from build123d import *

# Parameters (mm, degrees)
BOSS_EXTRUDE1_DEPTH = 6


with BuildPart() as part:
    # Sketch1 → Boss-Extrude1 (new body)
    with BuildSketch(Plane(origin=(330, 0, 0), x_dir=(0, 0, -1), z_dir=(1, 0, 0))):
        Polygon((-52.75, 244), (-52.75, 250), (-78.625, 250), (-78.625, 244), (-105, 244), (-105, 6), (-78.625, 6), (-78.625, 0), (-52.75, 0), (-52.75, 6), (-25.875, 6), (-25.875, 0), (0, 0), (0, 22.272727273), (-6, 22.272727273), (-6, 45.545454545), (0, 45.545454545), (0, 67.818181818), (-6, 67.818181818), (-6, 91.090909091), (0, 91.090909091), (0, 113.363636364), (-6, 113.363636364), (-6, 136.636363636), (0, 136.636363636), (0, 158.909090909), (-6, 158.909090909), (-6, 182.181818182), (0, 182.181818182), (0, 204.454545455), (-6, 204.454545455), (-6, 227.727272727), (0, 227.727272727), (0, 250), (-25.875, 250), (-25.875, 244), align=None)
    extrude(amount=-BOSS_EXTRUDE1_DEPTH)


solid = part.part
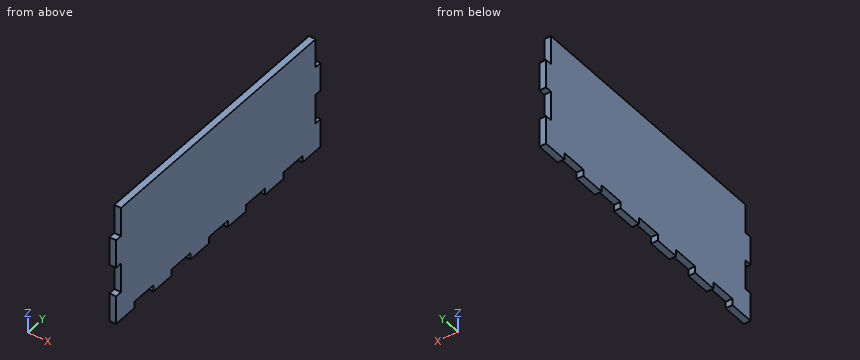
The model under review builds one solid part; all positions refer to its coordinate system, in mm. Give positions to 0.01 mm unless a question says otherwise; leave off trailing zeros. Write each loop counter-clockwise with the first axis right and the second up, starting at its lowest first coordinate (ties: lowest second). Pieces come first, ordered by that corner, then holes. Notation, with made-up numbers: M 21.5,5.25 L 50.5,5.25 A36 cw 50.5,39.25 Z; hole C -28,4 d11. An arc over 180 degrees is marked long. One line per question, with ' | ' between items. Start each with the question number.
Item 1: Wall thickness on line 1 (Z direction, x = 326.55, y = 31); line 2 (Y direction, x = 326.9, z = 46.5): over which ranges is each line inside the solid? List them lowest first. Write a range as from..to.
Item 2: For pin 1 (3 mm diameter, centred on x = 326.5, y = 76.5, fed in from -Z); pin 2 (3 mm diameter, centred on x = 326, y = 4, fed in from +Z) (3 decimals), all flat-tipped, find the tip position at first contact; note any pin that passes through.
Item 3: We need section B-B on y = 225.5. Write out the cut boundary in (x, z).
Item 4: We need section A-A on z = 42. Write out the cut boundary in (x, y), plus the area to 3 significant figures.
Results found:
1) line 1: z = 6..105 | line 2: y = 6..244
2) pin 1: stops at z = 6 | pin 2: stops at z = 78.625
3) outline: M 324,6 L 330,6 L 330,105 L 324,105 Z
4) outline: M 324,6 L 330,6 L 330,244 L 324,244 Z | area: 1,430 mm2
